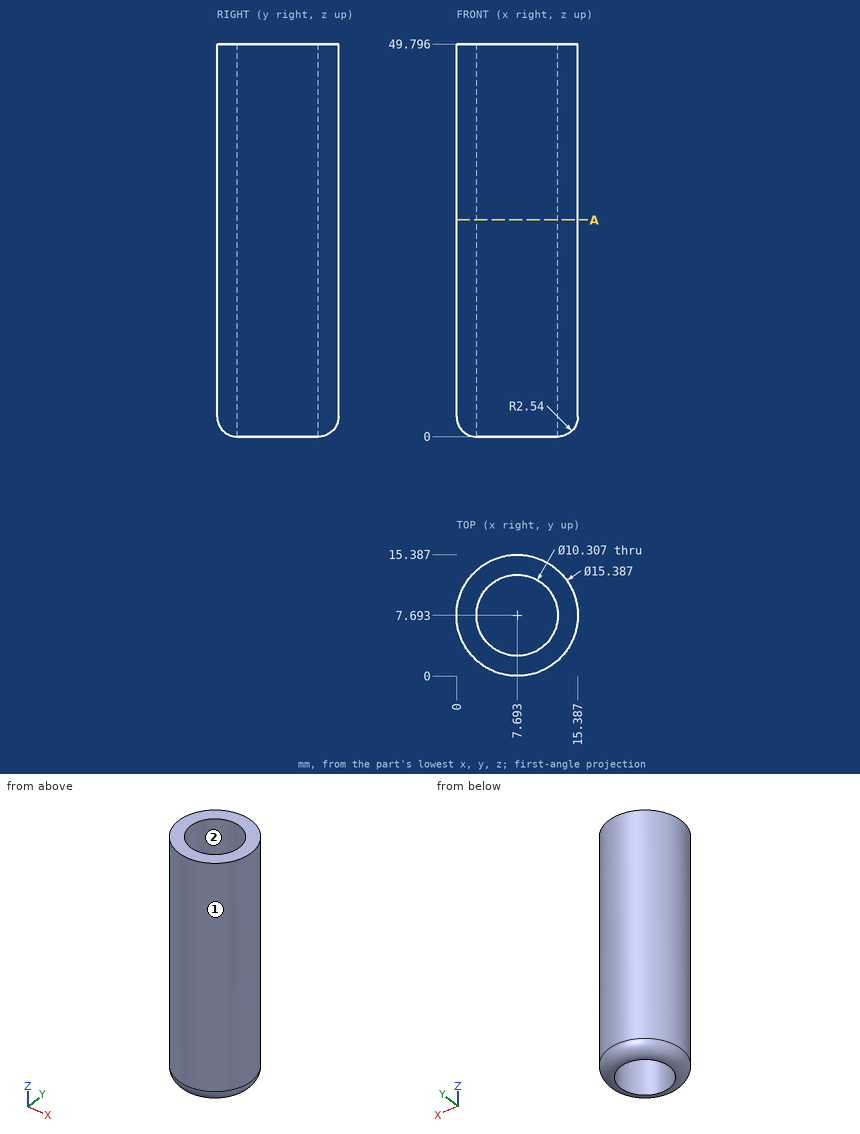
For this review, use the dimensioned drawing (mm, ordinates from the lowest corner) and the shaded views. Round coordinates to 2 decimals unless told otherwise and drop trailing zeros. Write each loop counter-clockwise with the first axis right and the second up, starting at its lowest first coordinate (ties: lowest second). Pieces come first, ordered by that corner, then holes. Notation, with made-up numbers: (-15, 4) -> (15, 4) arc R17 cw to (15, 19) -> close; hole circle Ø11 at (11.25, 76). An arc over 180 degrees is marked (long way). One line per item, written item: value. Start each with the question number.
Q1. The part is to be moulded in two halves that separate along Y. For the marked faces 1 and 2, say which applies: pulls with the +Y half, pulls with the -Y half, needs draft (parallel to the pull), parting line crosses it, or undercut.
Q2. Add section A-A (z = 27.5). Give the boundary of the cut face in (x, y).
Q3. To check wall thickness, follow probe 1 along X at (y, z) = (7.75, 17); probe 2 along Z at (x, y) = (12.5, 10); probe 3 along X at (y, z) = (3.25, 36) (1 decimal). State the ranges of each line that lie inside material, in increasing order.
Q4. Insertion check: P1, Ø1, axis at y = 6.5, z = 8.5, coming from the -X side; P2, Ø1, axis at x = 5, z = 37, coming from the +Y side; P3, Ø1.5, axis at x = 9, z = 13, coming from the -Y side. Each pin has a flat end and moves straight along its axis. Give the tip position at first contact, or say it passes through.
Response:
1. face 1: parting line crosses it
1. face 2: undercut
2. outline: circle Ø15.39 at (7.69, 7.69); hole circle Ø10.31 at (7.69, 7.69)
3. probe 1: x = 0 to 2.54, 12.85 to 15.39
3. probe 2: z = 0.01 to 49.8
3. probe 3: x = 1.4 to 5.1, 10.3 to 14
4. P1: stops at x = 0.03
4. P2: stops at y = 15.07
4. P3: stops at y = 0.02
